Autodesk Inventor part; units mm, degrees
ref_plane "YZ Plane" through (0, 0, 0) normal (1, 0, 0) x (0, 1, 0)
ref_plane "XZ Plane" through (0, 0, 0) normal (0, 1, 0) x (-1, 0, 0)
ref_plane "XY Plane" through (0, 0, 0) normal (0, 0, 1) x (1, 0, 0)
sketch "Skizze1" plane through (0, 0, 0) normal (0, 1, 0) x (-1, 0, 0)
  line L0 (0, 0) -> (1.3, 0)
  line L1 (1.3, 0) -> (1.3, -21.5)
  line L2 (1.3, -21.5) -> (0, -21.5)
  line L3 (0, -21.5) -> (0, 0)
  line L4 (1.3, 0) -> (2.8, 0)
  line L5 (2.8, 0) -> (2.8, -21.5)
  line L6 (2.8, -21.5) -> (1.3, -21.5)
  line L7 (1.3, -21.5) -> (1.3, 0)
  line L8 (2.8, 0) -> (1.3, 0)
  line L9 (1.3, 0) -> (1.3, -2)
  line L10 (1.3, -2) -> (2.8, -2)
  line L11 (2.8, -2) -> (2.8, 0)
  line L12 (1.3, -21.5) -> (2.8, -21.5)
  line L13 (2.8, -21.5) -> (2.8, -19.5)
  line L14 (2.8, -19.5) -> (1.3, -19.5)
  line L15 (1.3, -19.5) -> (1.3, -21.5)
  point P0 (1.3, -19.5)
  point P1 (2.8, -2)
  point P2 (1.3, -2)
  dimension "d0" = 1.3
  dimension "d1" = 21.5
  dimension "d2" = 1.5
  dimension "d3" = 2
  dimension "d4" = 2
extrude "Extrusion1" add sketch "Skizze1" along normal blind 10 contours L0 L1 L2 L3 | L10 L5 L14 L1
sketch "Skizze3" plane through (-2.8, 0, -19.5) normal (-1, 0, 0) x (0, 0, 1)
  line L0 (12.2393, 3.0088) -> (12.2393, 2.4088)
  line L1 (12.2393, 2.4088) -> (10.2953, 2.4088)
  arc A0 (9.9169, 2.6153) -> (10.2953, 2.4088) centre (10.2953, 2.8588) ccw
  line L2 (9.9169, 2.6153) -> (8.6983, 4.5088)
  line L3 (8.6983, 4.5088) -> (15.3893, 4.5088)
  line L4 (15.3893, 4.5088) -> (15.3893, 3.9088)
  line L5 (15.3893, 3.9088) -> (16.9481, 4.8088)
  line L6 (16.9481, 4.8088) -> (15.3893, 5.7088)
  line L7 (15.3893, 5.7088) -> (15.3893, 5.1088)
  line L8 (15.3893, 5.1088) -> (6.148, 5.1088)
  line L9 (6.148, 5.1088) -> (7.3604, 7.0016)
  arc A1 (7.7393, 7.2088) -> (7.3604, 7.0016) centre (7.7393, 6.7588) ccw
  line L10 (7.7393, 7.2088) -> (10.0408, 7.2088)
  arc A2 (10.0408, 7.2088) -> (10.0408, 7.8088) centre (10.8893, 7.5088) ccw
  line L11 (10.0408, 7.8088) -> (7.7393, 7.8088)
  arc A3 (7.7393, 7.8088) -> (6.8551, 7.3252) centre (7.7393, 6.7588) ccw
  line L12 (6.8551, 7.3252) -> (5.5682, 5.3161)
  arc A4 (5.1893, 5.1088) -> (5.5682, 5.3161) centre (5.1893, 5.5588) ccw
  line L13 (5.1893, 5.1088) -> (3.959, 5.1088)
  arc A5 (3.959, 5.1088) -> (3.959, 4.5088) centre (2.4893, 4.8088) ccw
  line L14 (3.959, 4.5088) -> (7.7393, 4.5088)
  arc A6 (8.1177, 4.3024) -> (7.7393, 4.5088) centre (7.7393, 4.0588) ccw
  line L15 (8.1177, 4.3024) -> (9.4123, 2.2906)
  arc A7 (9.4123, 2.2906) -> (10.2953, 1.8088) centre (10.2953, 2.8588) ccw
  line L16 (10.2953, 1.8088) -> (12.2393, 1.8088)
  line L17 (12.2393, 1.8088) -> (12.2393, 1.2088)
  line L18 (12.2393, 1.2088) -> (14.0393, 1.2088)
  line L19 (14.0393, 1.2088) -> (14.0393, 3.0088)
  line L20 (14.0393, 3.0088) -> (12.2393, 3.0088)
  point P0 (19.5, 0)
  point P1 (8.1177, 4.3024)
  point P2 (9.4123, 2.2906)
  point P3 (10.2953, 1.8088)
  point P4 (9.9169, 2.6153)
  point P5 (6.148, 5.1088)
  point P6 (7.3604, 7.0016)
  point P7 (7.7393, 7.2088)
  point P8 (10.0408, 7.8088)
  point P9 (7.7393, 7.8088)
  point P10 (6.8551, 7.3252)
  point P11 (5.1893, 5.1088)
  point P12 (3.959, 5.1088)
  point P13 (3.959, 4.5088)
  point P14 (7.7393, 4.5088)
extrude "Extrusion2" add sketch "Skizze3" along normal blind 0.4
sketch "Skizze4" plane through (-2.8, 0, -2) normal (0, 0, 1) x (1, 0, 0)
  line L0 (1.5, 10) -> (0, 10)
  line L1 (0, 10) -> (-1.5, 10)
  line L2 (0, 10) -> (-1.5, 10)
  line L3 (-1.5, 10) -> (-1.5, 9.5)
  line L4 (-1.5, 9.5) -> (0, 9.5)
  line L5 (0, 9.5) -> (0, 10)
  line L6 (0, 9.5) -> (0, 8)
  line L7 (0, 7.8088) -> (-0.4, 7.8088)
  line L8 (-1.5, 9.5) -> (0, 9.5) construction
  line L9 (0, 9.5) -> (0, 7.8088) construction
  line L10 (0, 0) -> (0, 10)
  spline S0 degree 2 poles (-1.5, 9.5) (0, 9.5) (0, 7.8088) knots 1 1 1 2 2 2
  point P0 (2.8, 0)
  dimension "d9" = 1.5
  dimension "d10" = 0.5
  dimension "d11" = 1.5
extrude "Extrusion3" add sketch "Skizze4" against normal up to surface (17.5 mm away)
sketch "Skizze5" plane through (-1.3, 0, -2) normal (-1, 0, 0) x (0, 0, 1)
  line L0 (0, 10) -> (2, 10)
  line L1 (2, 10) -> (2, 2)
  line L2 (2, 0) -> (2, 10)
  line L3 (2, 2) -> (-19.5, 2)
  line L4 (-19.5, 0) -> (-19.5, 10)
  circle A0 centre (2, 2) radius 1.25
  circle A1 centre (-19.5, 2) radius 1.25
  line L5 (2, 0) -> (-19.5, 0)
  line L6 (1, 0) -> (2, 2)
  line L7 (-19.5, 0) -> (-17.5, 0)
  line L8 (-18.5, 0) -> (-19.5, 2)
  point P0 (1.441, 0.882)
  point P1 (2, 0.75)
  point P2 (-18.5, 0)
  point P3 (-18.941, 0.882)
  point P4 (-19.5, 0.75)
  dimension "d14" = 8
  dimension "d15" = 2.5
  dimension "d16" = 2.5
extrude "Extrusion4" cut sketch "Skizze5" against normal up to surface (1.3 mm away) contours A0 L2 L1 | L1 L3 A0 | L6 A0 L3 | L2 A0 L6 | L2 L5 L6 A0 | A1 L8 L3 | L3 L4 A1 | L8 A1 L4 | L4 A1 | L8 L5 L4 A1
fillet "Rundung1" radius 0.3 4 edges at (-1.3, 6.625, 0) (-1.3, 6.625, -21.5) (0, 6.625, -21.5) (0, 6.625, 0)
properties part number "USB-Deckel"
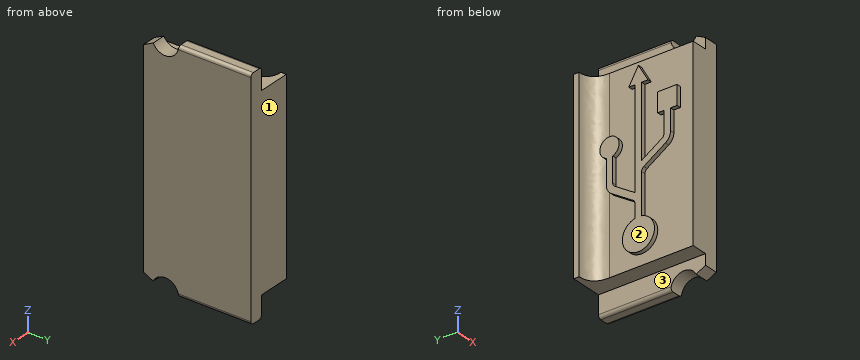
Geometry: final body of the model. Coordinates: model frame, mm. Face numbers are marked on the shaded views. A direction names the side the tool comes from. Coordinates: 2 decimals unless noted, no trailing zeros. Order: outer loops, then holes, each group sorted by start corner. A loop starts at its lowest first (then second) coordinate and runs counter-clockwise, first axis right, second up.
(1) Section query D-D (y = 6). Return the cut outline in (x, z).
(2) Section query A-A (y = 9.75). Return the cut outline in (x, z).
(3) Section query B-B (x = -2). Return the cut outline in (y, z), plus the area to 3 significant figures.
(4) Section query C-C (y = 1.5). Return the cut outline in (x, z), plus the area to 3 significant figures.
(5) Access query for the marked faces 1, 2 and 3. Directions: +Z, -Z, +X, -X, +Y, -Y. A direction counts if a zero-diameter tool reaches every point of the face in a straight line with its end or side. Return the directions, or none.
(6) First-contact query: pin 1 (1.9 mm diameter, centred on y = 7.5, z = -1, fed in from -X); pin 2 (4 mm diameter, centred on y = 5.5, z = -14, fed in from -X); pin 3 (1 mm diameter, centred on x = -2.5, y = 8.5, fed in from -Z). Flat tips, straight axial feed; report the tip coordinate or a pass-through.
(7) Material intervals for probe 1 along Z at (x, y) = (-2.7, 3); probe 2 along X at (y, z) = (0.5, -5.25); probe 3 along X at (y, z) = (7.25, -20.5), sorted ascending.
Solution:
1. outline: (-3.2, -17.92) - (-2.8, -17.92) - (-2.8, -19.5) - (-1.3, -19.5) - (-1.3, -21.2) arc R0.3 ccw to (-1, -21.5) - (-0.3, -21.5) arc R0.3 ccw to (0, -21.2) - (0, -0.3) arc R0.3 ccw to (-0.3, 0) - (-1, 0) arc R0.3 ccw to (-1.3, -0.3) - (-1.3, -2) - (-2.8, -2) - (-2.8, -12.78) - (-3.2, -12.78) - (-3.2, -13.49) - (-2.8, -13.49) - (-2.8, -16.1) - (-3.2, -16.1) - close
2. outline: (-4.3, -19.5) - (-1.3, -19.5) - (-1.3, -21.2) arc R0.3 ccw to (-1, -21.5) - (-0.3, -21.5) arc R0.3 ccw to (0, -21.2) - (0, -0.3) arc R0.3 ccw to (-0.3, 0) - (-1, 0) arc R0.3 ccw to (-1.3, -0.3) - (-1.3, -2) - (-4.3, -2) - close
3. outline: (0, -19.5) - (10, -19.5) - (10, -2) - (0, -2) - close
3. area: 175 mm2
4. outline: (-3.2, -7.26) - (-2.8, -7.26) - (-2.8, -19.5) - (-1.3, -19.5) - (-1.3, -20.35) - (0, -20.35) - (0, -1.15) - (-1.3, -1.15) - (-1.3, -2) - (-2.8, -2) - (-2.8, -5.46) - (-3.2, -5.46) - close
4. area: 51.9 mm2
5. face 1: +Z, -Z, +X, -X, +Y
5. face 2: +Z, -Z, -X, -Y
5. face 3: -Z, -X, +Y, -Y
6. pin 1: stops at x = -1.3
6. pin 2: stops at x = -3.2
6. pin 3: stops at z = -19.5
7. probe 1: z = -19.5 to -2
7. probe 2: x = -2.8 to 0
7. probe 3: x = -1.3 to 0
